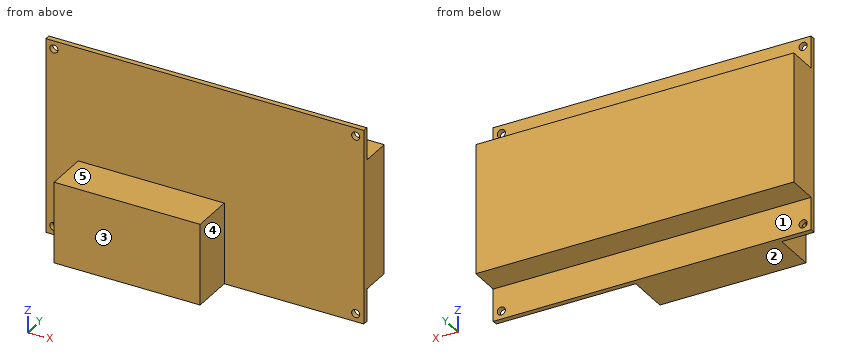
```python
from build123d import *

# Parameters (mm, degrees)
SKETCH_1_W          = 98
SKETCH_1_H          = 10
SKETCH_1_H_2        = 40
EXTRUDE_1_DEPTH     = 1.6
SKETCH_1_4_W        = 98
SKETCH_1_4_H        = 40
EXTRUDE_2_DEPTH     = 11
SKETCH_2_W          = 45
SKETCH_2_H          = 25
EXTRUDE_3_DEPTH     = 13
CUT_EXTRUDE_1_REACH = 13
SKETCH_3_R          = 1.25


with BuildPart() as part:
    # Sketch 1 → Extrude 1 (new body)
    with BuildSketch(Plane(origin=(0, 0, 0), x_dir=(1, 0, 0), z_dir=(0, 1, 0))):
        with Locations((0, 25)):
            Rectangle(SKETCH_1_W, SKETCH_1_H)
        Rectangle(SKETCH_1_W, SKETCH_1_H_2)
        with Locations((0, -25)):
            Rectangle(SKETCH_1_W, SKETCH_1_H)
    extrude(amount=EXTRUDE_1_DEPTH)

    # Sketch 1_4 → Extrude 2 (add)
    with BuildSketch(Plane(origin=(0, 0, 0), x_dir=(1, 0, 0), z_dir=(0, 1, 0))):
        Rectangle(SKETCH_1_4_W, SKETCH_1_4_H)
    extrude(amount=EXTRUDE_2_DEPTH)

    # Sketch 2 → Extrude 3 (add)
    with BuildSketch(Plane.XZ):
        with Locations((-16.5, -17.5)):
            Rectangle(SKETCH_2_W, SKETCH_2_H)
    extrude(amount=EXTRUDE_3_DEPTH)

    # Sketch 3 → Cut-Extrude 1 (cut, up to next)
    with BuildSketch(Plane.XZ, mode=Mode.PRIVATE) as cut_extrude_1_sk1:
        with Locations((46.5, 27.5)):
            Circle(SKETCH_3_R)
    cut_extrude_1_tool1 = extrude(cut_extrude_1_sk1.sketch, amount=-CUT_EXTRUDE_1_REACH, mode=Mode.PRIVATE) & part.part
    add(cut_extrude_1_tool1.solids().sort_by_distance((46.5, 0, 27.5))[0], mode=Mode.SUBTRACT)
    # Sketch 3 → Cut-Extrude 1 (cut, up to next)
    with BuildSketch(Plane.XZ, mode=Mode.PRIVATE) as cut_extrude_1_sk2:
        with Locations((-46.5, 27.5)):
            Circle(SKETCH_3_R)
    cut_extrude_1_tool2 = extrude(cut_extrude_1_sk2.sketch, amount=-CUT_EXTRUDE_1_REACH, mode=Mode.PRIVATE) & part.part
    add(cut_extrude_1_tool2.solids().sort_by_distance((-46.5, 0, 27.5))[0], mode=Mode.SUBTRACT)
    # Sketch 3 → Cut-Extrude 1 (cut, up to next)
    with BuildSketch(Plane.XZ, mode=Mode.PRIVATE) as cut_extrude_1_sk3:
        with Locations((-46.5, -27.5)):
            Circle(SKETCH_3_R)
    cut_extrude_1_tool3 = extrude(cut_extrude_1_sk3.sketch, amount=-CUT_EXTRUDE_1_REACH, mode=Mode.PRIVATE) & part.part
    add(cut_extrude_1_tool3.solids().sort_by_distance((-46.5, 0, -27.5))[0], mode=Mode.SUBTRACT)
    # Sketch 3 → Cut-Extrude 1 (cut, up to next)
    with BuildSketch(Plane.XZ, mode=Mode.PRIVATE) as cut_extrude_1_sk4:
        with Locations((46.5, -27.5)):
            Circle(SKETCH_3_R)
    cut_extrude_1_tool4 = extrude(cut_extrude_1_sk4.sketch, amount=-CUT_EXTRUDE_1_REACH, mode=Mode.PRIVATE) & part.part
    add(cut_extrude_1_tool4.solids().sort_by_distance((46.5, 0, -27.5))[0], mode=Mode.SUBTRACT)


solid = part.part
```
Read the model definition and answer for the solid it produces. Units are mm, in the model's axes. Face numbers are marked on the shaded views. A direction names the side the tool comes from. Give positions to 0.01 mm unless a question says otherwise; leave off trailing zeros. Write each loop counter-clockwise with the first axis right and the second up, starting at its lowest first coordinate (ties: lowest second). Pieces come first, ordered by that corner, then holes. Notation, with made-up numbers: (54.25, 51.5) -> (94.25, 51.5) arc R18 cw to (94.25, 58.5) -> close; hole circle Ø2 at (-28, 53.5). An arc over 180 degrees is marked (long way). Answer as a JSON object with one key per item and string values.
1) Section B-B on x = -46.5 is taken. Write down the section's boundary in (y, z), then the cut area to 3 significant figures.
Findings below:
{"outline": "(0, -30) -> (1.6, -30) -> (1.6, -28.75) -> (0, -28.75) -> close; (0, -26.25) -> (1.6, -26.25) -> (1.6, -20) -> (11, -20) -> (11, 20) -> (1.6, 20) -> (1.6, 26.25) -> (0, 26.25) -> close; (0, 28.75) -> (1.6, 28.75) -> (1.6, 30) -> (0, 30) -> close", "area": "464 mm^2"}
2) Section C-C on x = 2 is taken. Write down the section's boundary in (y, z).
Findings below:
{"outline": "(-13, -30) -> (1.6, -30) -> (1.6, -20) -> (11, -20) -> (11, 20) -> (1.6, 20) -> (1.6, 30) -> (0, 30) -> (0, -5) -> (-13, -5) -> close"}
3) Straight lines are drawn through the part: probe 1 along Z at (x, y) = (-46.5, 0.8); probe 2 along Y at (x, z) = (36, -6.5); probe 3 along Y at (x, z) = (-15, 26). For each, find the intervals that lie inside material, in ascending order. Write a range as from..to.
Findings below:
{"probe 1": "z = -30..-28.75, -26.25..26.25, 28.75..30", "probe 2": "y = 0..11", "probe 3": "y = 0..1.6"}
4) Section D-D on z = -16 is taken. Write down the section's boundary in (x, y).
Findings below:
{"outline": "(-49, 0) -> (-39, 0) -> (-39, -13) -> (6, -13) -> (6, 0) -> (49, 0) -> (49, 11) -> (-49, 11) -> close"}
5) Flat-ended cylindrical pins translate along their axes: pin 1 Ø3 at (x, z) = (-46.5, -27.5) entering from +Y; pin 2 Ø2 at (x, z) = (46.5, 27.5) entering from -Y; pin 3 Ø7.5 at (x, y) = (-22, 8) entering from -Z; pin 4 Ø3 at (x, y) = (-18.5, 8.5) entering from +Z. Find the tip coordinate at first contact, or state that the pin passes through.
Findings below:
{"pin 1": "stops at y = 1.6", "pin 2": "passes through", "pin 3": "stops at z = -20", "pin 4": "stops at z = 20"}
6) Section A-A on z = -27.5 is taken. Write down the section's boundary in (x, y), then the cut area to 3 significant figures.
Findings below:
{"outline": "(-49, 0) -> (-47.75, 0) -> (-47.75, 1.6) -> (-49, 1.6) -> close; (-45.25, 0) -> (-39, 0) -> (-39, -13) -> (6, -13) -> (6, 0) -> (45.25, 0) -> (45.25, 1.6) -> (-45.25, 1.6) -> close; (47.75, 0) -> (49, 0) -> (49, 1.6) -> (47.75, 1.6) -> close", "area": "734 mm^2"}
7) A tool of negligible diameter and unlimited length cuts with its end or side. For the marked faces 1, 2, 3, 4 and 5, from which of +Z, -Z, +X, -X, +Y, -Y can it reach the whole face along a straight path? Write none if from no direction.
Findings below:
{"face 1": "-Z, +X, -X, +Y", "face 2": "-Z, +X, -X, +Y, -Y", "face 3": "+Z, -Z, +X, -X, -Y", "face 4": "+Z, -Z, +X, -Y", "face 5": "+Z, +X, -X, -Y"}
